from build123d import *

# Parameters (mm, degrees)
SKETCH_2_R          = 1
CUT_EXTRUDE_1_DEPTH = 5


with BuildPart() as part:
    # 草图1 → 旋转1 (revolve)
    with BuildSketch(Plane.XY):
        Polygon((-33.409090909, 0), (18.570909091, 0), (18.570909091, 3), (-1.429090909, 3), (-1.429090909, 3.5), (-11.429090909, 3.5), (-11.429090909, 3.95), (-13.509090909, 3.95), (-13.509090909, 3.75), (-14.409090909, 3.75), (-14.409090909, 3.95), (-31.409090909, 3.95), (-31.409090909, 4.5), (-33.409090909, 4.5), align=None)
    revolve(axis=Axis((-66.136363636, 0, 0), (1, 0, 0)))

    # 草图2 → 切除-拉伸1 (cut, symmetric)
    with BuildSketch(Plane(origin=(0, 0, 0), x_dir=(1, 0, 0), z_dir=(0, 1, 0))):
        with Locations((11.570909091, 0)):
            Circle(SKETCH_2_R)
    extrude(amount=CUT_EXTRUDE_1_DEPTH, both=True, mode=Mode.SUBTRACT)


solid = part.part
For this review, take the finished solid that the model builds, in its own axes (mm). A direction names the side the tool comes from. Give positions to 0.01 mm unless a question says otherwise; leave off trailing zeros. Order: outer loops, then holes, each group sorted by start corner. A loop starts at its lowest first (then second) coordinate and runs counter-clockwise, first axis right, second up. Notation, with made-up numbers: M -33,-8.75 L 20,-8.75 A26 ccw 20,28.25 Z; hole C 37,-33 d10. An arc over 180 degrees is marked long. Answer in a Markdown table with one row per item. Add a question column.
(1) Consider section C-C on y = -2. State the section outline as (x, z) points.
(2) Wall thickness on probe 1 along X at (y, z) = (0.5, 3.75); probe 2 along X at (y, z) = (-0.25, 0); probe 3 along Y at (x, z) = (8, 0.25): over which ranges is each line inside the solid? List them lowest first. Write a range as [from, to].
(3) For pin 1 (2 mm diameter, centred on x = -6, z = -3, fed in from +Y); pin 2 (2 mm diameter, centred on x = 12.5, y = 1.5, fed in from -Z); pin 3 (1.8 mm diameter, centred on x = 11.57, z = 0, fed in from -Y); pin 4 (4 mm diameter, centred on x = -15.5, y = 0.5, fed in from -Z), all flat-tipped, find the tip position at first contact; note any pin that passes through.
(4) For faces 1 (the face through (-33.409, 0, 0)), 2 (the face through (8.43, 2.77, -1.15)), 3 (the face through (-13.965, -3.746, 0.165)), list the 3-axis set-ups (+Z, -Z, +X, -X, +Y, -Y) from which the entire face can be reached by the end or side of a thin tool; tool diameter is ignored.
(5) Mouldability with a two-part tool opening along X and no side actions: class faces 4 (the face through (-31.409, -3, -3)), 5 (the face through (10.57, 0.04, -0.04)), 6 (the face through (-32.42, -0.59, 4.46)) as +X half, -X half, draft (parallel to the pull), parting line (faces both ways), or undercut.
(6) Consider section A-A on z = 0. State the section outline as (x, y) points, and give its area (3 significant figures).
(7) Consider section D-D on x = -22. State the section outline as (y, z) points.
(8) Consider section B-B on y = 1.25. State the section outline as (x, z) points.
Evaluation:
| question | item | result |
|---|---|---|
| 1 | outline | M -33.41,-4.03 L -31.41,-4.03 L -31.41,-3.41 L -14.41,-3.41 L -14.41,-3.17 L -13.51,-3.17 L -13.51,-3.41 L -11.43,-3.41 L -11.43,-2.87 L -1.43,-2.87 L -1.43,-2.24 L 18.57,-2.24 L 18.57,2.24 L -1.43,2.24 L -1.43,2.87 L -11.43,2.87 L -11.43,3.41 L -13.51,3.41 L -13.51,3.17 L -14.41,3.17 L -14.41,3.41 L -31.41,3.41 L -31.41,4.03 L -33.41,4.03 Z; hole C 11.57,0 d2 |
| 2 | probe 1 | x = [-33.41, -14.41], [-13.51, -11.43] |
| 2 | probe 2 | x = [-33.41, 10.57], [12.57, 18.57] |
| 2 | probe 3 | y = [-2.99, 2.99] |
| 3 | pin 1 | stops at y = 2.87 |
| 3 | pin 2 | stops at z = -2.96 |
| 3 | pin 3 | passes through |
| 3 | pin 4 | stops at z = -3.95 |
| 4 | face 1 | +Z, -Z, -X, +Y, -Y |
| 4 | face 2 | +X |
| 4 | face 3 | none |
| 5 | face 4 | +X half |
| 5 | face 5 | undercut |
| 5 | face 6 | draft |
| 6 | outline | M -33.41,-4.5 L -31.41,-4.5 L -31.41,-3.95 L -14.41,-3.95 L -14.41,-3.75 L -13.51,-3.75 L -13.51,-3.95 L -11.43,-3.95 L -11.43,-3.5 L -1.43,-3.5 L -1.43,-3 L 10.57,-3 L 10.57,3 L -1.43,3 L -1.43,3.5 L -11.43,3.5 L -11.43,3.95 L -13.51,3.95 L -13.51,3.75 L -14.41,3.75 L -14.41,3.95 L -31.41,3.95 L -31.41,4.5 L -33.41,4.5 Z; M 12.57,-3 L 18.57,-3 L 18.57,3 L 12.57,3 Z |
| 6 | area | 353 mm^2 |
| 7 | outline | C 0,0 d7.9 |
| 8 | outline | M -33.41,-4.32 L -31.41,-4.32 L -31.41,-3.75 L -14.41,-3.75 L -14.41,-3.54 L -13.51,-3.54 L -13.51,-3.75 L -11.43,-3.75 L -11.43,-3.27 L -1.43,-3.27 L -1.43,-2.73 L 18.57,-2.73 L 18.57,2.73 L -1.43,2.73 L -1.43,3.27 L -11.43,3.27 L -11.43,3.75 L -13.51,3.75 L -13.51,3.54 L -14.41,3.54 L -14.41,3.75 L -31.41,3.75 L -31.41,4.32 L -33.41,4.32 Z; hole C 11.57,0 d2 |
